Geometry check sheet. Reference: the model listing, model coordinates, mm. Round coordinates to 2 decimals unless told otherwise and drop trailing zeros. Order: outer loops, then holes, each group sorted by start corner. A loop starts at its lowest first (then second) coordinate and runs counter-clockwise, first axis right, second up. Notation, with made-up numbers: (-39.5, 39) - (-1.5, 39) arc R6 ccw to (-1.5, 45) - close; hole circle Ø3 at (2, 10.25). An arc over 180 degrees is marked (long way). Return JSON: item names as keys, results as strings. Group by question number.
Q1. Sectioned sample at C-C, the plane y = -2.5. Record the cut outline in (x, z) (3 decimals).
Q2. Sectioned sample at A-A, the plane z = -20. Record the cut outline in (x, y), then the cut area to 3 significant figures.
Q3. Gauge pin test, flat end, axial feed: pin 1 Ø3 at (y, z) = (-5, -67.5) entering from -X. Record the tip position at first contact, or that the pin passes through.
Q4. Draft check along X on faces 1 (the flat face through (13, 0, -40)), 2 (the flat face through (44.45, -3, -42)), 3 (the cylindrical face through (38.24, -3.13, 6.35)). Enter one of: pulls with the +X half, pulls with the -X half, needs draft (parallel to the pull), parting line crosses it, or undercut.
Q5. Material ranges on line 1 along X through (y, z) = (-5.25, -55); line 2 along X through (y, z) = (-4, -12.5); line 3 along X through (y, z) = (-1, -8), recorded low to high.
Q6. Sectioned sample at D-D, the plane z = -75.5. Record the cut outline in (x, y).
Q7. Sectioned sample at B-B, the plane x = -38.1. Record the cut outline in (y, z) (3 decimals), then the cut area to 3 significant figures.
```python
from build123d import *

# Parameters (mm, degrees)
F1_DEPTH = 6.35
F2_D     = 6.35


# Not quite as in the source:
# - a feature names something its author has since deleted; it is built from what else it names


with BuildPart() as f1:
    # F0 (on Front) → F1 (new body)
    with BuildSketch(Plane.XZ):
        with BuildLine():
            ThreePointArc((44.45, 0), (38.1, 6.35), (31.75, 0))
            ThreePointArc((31.75, 0), (38.1, -6.35), (44.45, 0))
        make_face()
        with BuildLine():
            Line((31.75, -31.1085197333), (31.75, 0))
            ThreePointArc((31.75, 0), (21.3576281747, -20.379309083), (0, -28.575))
            ThreePointArc((0, -28.575), (-21.3576281747, -20.379309083), (-31.75, 0))
            ThreePointArc((-31.75, 0), (-38.1, -6.35), (-44.45, 0))
            ThreePointArc((-44.45, 0), (-31.4308964237, -31.4308964237), (0, -44.45))
            ThreePointArc((0, -44.45), (9.7634350172, -43.3644766677), (19.05, -40.1609262841))
            ThreePointArc((19.05, -40.1609262841), (25.8001262805, -36.1960769132), (31.75, -31.1085197333))
        make_face()
        with BuildLine():
            ThreePointArc((44.45, 0), (38.1, -6.35), (31.75, 0))
            Line((31.75, 0), (31.75, -31.1085197333))
            ThreePointArc((31.75, -31.1085197333), (41.1527034349, -16.8005208253), (44.45, 0))
        make_face()
        with BuildLine():
            ThreePointArc((-44.45, 0), (-38.1, -6.35), (-31.75, 0))
            ThreePointArc((-31.75, 0), (-38.1, 6.35), (-44.45, 0))
        make_face()
        with BuildLine():
            Line((44.45, -44.45), (44.45, 0))
            ThreePointArc((44.45, 0), (41.1527034349, -16.8005208253), (31.75, -31.1085197333))
            Line((31.75, -31.1085197333), (31.75, -44.45))
            Line((31.75, -44.45), (44.45, -44.45))
        make_face()
        with BuildLine():
            Line((31.75, -44.45), (31.75, -31.1085197333))
            ThreePointArc((31.75, -31.1085197333), (25.8001262805, -36.1960769132), (19.05, -40.1609262841))
            Line((19.05, -40.1609262841), (19.05, -44.45))
            Line((19.05, -44.45), (31.75, -44.45))
        make_face()
        with BuildLine():
            Line((44.45, -82.55), (44.45, -44.45))
            Line((44.45, -44.45), (31.75, -44.45))
            Line((31.75, -44.45), (31.75, -69.85))
            ThreePointArc((31.75, -69.85), (40.7302561211, -73.5697438789), (44.45, -82.55))
        make_face()
        with BuildLine():
            Line((31.75, -69.85), (31.75, -44.45))
            Line((31.75, -44.45), (19.05, -44.45))
            Line((19.05, -44.45), (19.05, -82.55))
            ThreePointArc((19.05, -82.55), (22.7697438789, -73.5697438789), (31.75, -69.85))
        make_face()
        with BuildLine():
            Line((31.75, -82.55), (44.45, -82.55))
            ThreePointArc((44.45, -82.55), (40.7302561211, -73.5697438789), (31.75, -69.85))
            Line((31.75, -69.85), (31.75, -82.55))
        make_face()
        with BuildLine():
            ThreePointArc((19.05, -82.55), (31.75, -95.25), (44.45, -82.55))
            Line((44.45, -82.55), (31.75, -82.55))
            Line((31.75, -82.55), (19.05, -82.55))
        make_face()
        with BuildLine():
            Line((31.75, -82.55), (31.75, -69.85))
            ThreePointArc((31.75, -69.85), (22.7697438789, -73.5697438789), (19.05, -82.55))
            Line((19.05, -82.55), (31.75, -82.55))
        make_face()
    extrude(amount=F1_DEPTH)

    # F2 (through all)
    with Locations(Plane(origin=(0, 0, 0), x_dir=(1, 0, 0), z_dir=(0, 1, 0))):
        with Locations((-38.1, 0), (38.1, 0), (31.75, 82.55)):
            Hole(F2_D / 2)


solid = f1.part
```
Reply:
{
 "1": {"outline": "(-44.45, 0) arc R44.45 ccw to (19.05, -40.161) - (19.05, -82.55) arc R12.7 ccw to (44.45, -82.55) - (44.45, 0) arc R6.35 ccw to (31.75, 0) arc R31.926 cw to (-31.75, 0) arc R6.35 ccw to start; hole circle Ø6.35 at (-38.1, 0); hole circle Ø6.35 at (31.75, -82.55); hole circle Ø6.35 at (38.1, 0)"},
 "2": {"outline": "(-39.7, -6.35) - (-21.77, -6.35) - (-21.77, 0) - (-39.7, 0) - close; (21.77, -6.35) - (44.45, -6.35) - (44.45, 0) - (21.77, 0) - close", "area": "258 mm^2"},
 "3": {"pin 1": "x = 19.05"},
 "4": {"face 1": "needs draft", "face 2": "pulls with the +X half", "face 3": "undercut"},
 "5": {"line 1": "19.05 to 44.45", "line 2": "-42.66 to -27.71, 27.71 to 44.45", "line 3": "-43.72 to -29.84, 29.84 to 44.45"},
 "6": {"outline": "(19.05, -6.35) - (44.45, -6.35) - (44.45, 0) - (19.05, 0) - close"},
 "7": {"outline": "(-6.35, -22.895) - (0, -22.895) - (0, -3.175) - (-6.35, -3.175) - close; (-6.35, 3.175) - (0, 3.175) - (0, 6.35) - (-6.35, 6.35) - close", "area": "145 mm^2"}
}
